```python
from build123d import *

# Parameters (mm, degrees)
F0_W     = 600
F0_H     = 240
F1_DEPTH = 660
F3_DEPTH = 450.001
F4_W     = 600
F4_H     = 150
F4_H_2   = 240
F5_DEPTH = 660.001
F6_W     = 660
F6_H     = 660
F6_W_2   = 600
F6_H_2   = 600
F7_DEPTH = 400
F8_W     = 630
F8_H     = 660
F9_DEPTH = 2


with BuildPart() as f1:
    # F0 (on Right) → F1 (new body)
    with BuildSketch(Plane.YZ):
        Polygon((0, 450), (0, 0), (30, 0), (30, 150), (630, 150), (630, 0), (660, 0), (660, 450), align=None)
        with Locations((330, 300)):
            Rectangle(F0_W, F0_H, mode=Mode.SUBTRACT)
    extrude(amount=F1_DEPTH)

    # F2 (on face) → F3 (cut, through all)
    with BuildSketch(Plane.XY.offset(450)):
        Polygon((30, 30), (630, 30), (630, 630), (385, 630), (30, 630), align=None)
    extrude(amount=-F3_DEPTH, mode=Mode.SUBTRACT)

    # F4 (on face) → F5 (cut, through all)
    with BuildSketch(Plane(origin=(0, 660, 0), x_dir=(-1, 0, 0), z_dir=(0, 1, 0))):
        with Locations((-330, 75)):
            Rectangle(F4_W, F4_H)
        with Locations((-330, 300)):
            Rectangle(F4_W, F4_H_2)
    extrude(amount=-F5_DEPTH, mode=Mode.SUBTRACT)

    # F6 (on face) → F7 (join)
    with BuildSketch(Plane.XY.offset(450)):
        with Locations((330, 330)):
            Rectangle(F6_W, F6_H)
        with Locations((330, 330)):
            Rectangle(F6_W_2, F6_H_2, mode=Mode.SUBTRACT)
    extrude(amount=F7_DEPTH)

    # F8 (on face) → F9 (join)
    with BuildSketch(Plane(origin=(0, 0, 420), x_dir=(1, 0, 0), z_dir=(0, 0, -1))):
        with Locations((315, -330)):
            Rectangle(F8_W, F8_H)
    extrude(amount=-F9_DEPTH)


solid = f1.part
```
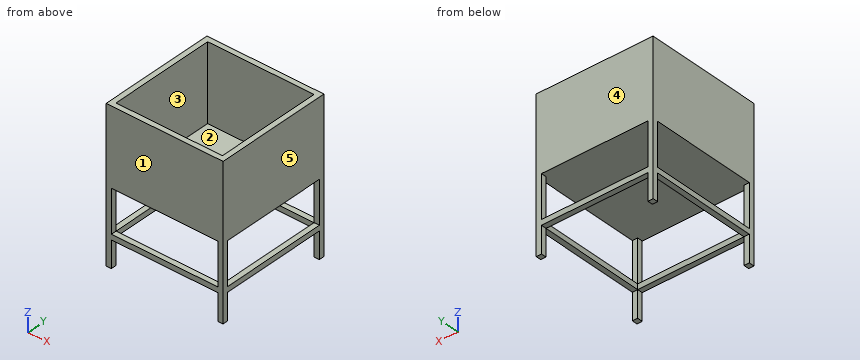
CAD build for the part. Positions are in the model's coordinates, mm. Face numbers are marked on the shaded views. A direction names the side the tool comes from. Round coordinates to 2 decimals unless told otherwise and drop trailing zeros. Write each loop counter-clockwise with the first axis right and the second up, starting at its lowest first coordinate (ties: lowest second). Pieces come first, ordered by that corner, then holes.
Item 1: Band-saw the part on B-B on z = 301.5. Write the cut outline in (x, y).
Filled in:
outline: (0, 0) - (30, 0) - (30, 30) - (0, 30) - close; (0, 630) - (30, 630) - (30, 660) - (0, 660) - close; (630, 0) - (660, 0) - (660, 30) - (630, 30) - close; (630, 630) - (660, 630) - (660, 660) - (630, 660) - close
Item 2: Tool access for the marked faces 1 and 2: list every direction of +Z, -Z, +X, -X, +Y, -Y with a clear straight run to the whole face (end or side of a thin tool).
Filled in:
face 1: +Z, -Z, +X, -X, -Y
face 2: +Z
Item 3: Drill centre lines: L1, parallel to X at y = 580, z = 646; L2, parallel to Z at x = 433, y = 190. Where is each one in solid material? Low to high.
Filled in:
L1: x = 0 to 30, 630 to 660
L2: z = 420 to 422
Item 4: Drop flat-ended pins along their axis: pin 1 Ø2 at (x, y) = (113, 195.5) entering from +Z; pin 2 Ø3 at (x, y) = (357, 565) entering from -Z. Give the stop position or say it passes through.
Filled in:
pin 1: stops at z = 422
pin 2: stops at z = 420
Item 5: Mould opens along Y. For the marked faces 3, 4 and 5 say: released by +Y, released by -Y, zero draft, split by the parting line, or undercut.
Filled in:
face 3: undercut
face 4: released by +Y
face 5: zero draft
Item 6: Band-saw the part on D-D on z = 786. Write the cut outline in (x, y).
Filled in:
outline: (0, 0) - (660, 0) - (660, 660) - (0, 660) - close; hole (30, 30) - (630, 30) - (630, 630) - (30, 630) - close
Item 7: Band-saw the part on A-A on x = 499.5. Write the cut outline in (y, z).
Filled in:
outline: (0, 150) - (30, 150) - (30, 180) - (0, 180) - close; (0, 420) - (660, 420) - (660, 850) - (630, 850) - (630, 422) - (30, 422) - (30, 850) - (0, 850) - close; (630, 150) - (660, 150) - (660, 180) - (630, 180) - close
